Here's how the part is built. I have some questions about the finished solid (model axes, mm). A direction names the side the tool comes from. Round coordinates to 2 decimals unless told otherwise and drop trailing zeros. Order: outer loops, then holes, each group sorted by start corner. A loop starts at its lowest first (then second) coordinate and runs counter-clockwise, first axis right, second up. Notation, with made-up numbers: (87.5, 73) -> (145.5, 73) arc R25 ccw to (145.5, 99) -> close; hole circle Ø1 at (43, 15). An arc over 180 degrees is marked (long way). Use a Markdown table: item, result. Add a question column.
(1) Thinking about a two-plate mould opening in X: for faces 6 (the face through (10, 19, 0)), 7 (the face through (0, 34, 20.25)), 8 (the face through (-0.6, 31, -23)), 9 (the face through (-5, 29, -22)), which applies, pulls with the +X half, pulls with the -X half, needs draft (parallel to the pull), parting line crosses it, or undercut?
(2) I want a section at A-A, the plane z = -24.25. Please give me the cut outline in (x, y), then the cut area to 3 significant figures.
(3) I'm going to push flat-ended pins straight in: P1, Ø0.6, axis at y = 30.5, z = -24.5, coming from the +X side; P2, Ø4, axis at y = 6, z = 23.5, coming from the +X side; P3, Ø4, axis at x = 0, z = 10.25, coming from the +Y side; P4, Ø5, axis at x = 4, z = -22, coming from the -Y side. Where does each tip first touch, or does it pass through?
(4) I want a section at C-C, the plane x = 0. Please give me the cut outline in (y, z), then the cut area to 3 significant figures.
(5) If I drill on probe 1 along X at (y, z) = (29, -24); probe 2 along Z at (x, y) = (5, 28.6); probe 3 along Y at (x, z) = (8.25, -20.5), over which ranges is the centre line in solid material (lowest first)?
(6) I want a section at B-B, the plane z = 10.25. Please give me the cut outline in (x, y).
(7) On a 3-axis mill with a long thin cutter (end or side, diameter ignored), from which of +Z, -Z, +X, -X, +Y, -Y can I reach the whole of each face in a straight line? I mean faces 1 (the face through (0, 8, 23)), 2 (the face through (0, 27.5, -24)), 3 (the face through (6, 30, 22)), 4 (the face through (-6, 30, -22)), 5 (the face through (-3.75, 6, 23)). Say none if no direction works.
(8) I want a section at D-D, the plane y = 31. Please give me the cut outline in (x, z), then the cut area to 3 significant figures.
Autodesk Inventor part; units mm, degrees
ref_plane "YZ Plane" through (0, 0, 0) normal (1, 0, 0) x (0, 1, 0)
ref_plane "XZ Plane" through (0, 0, 0) normal (0, 1, 0) x (-1, 0, 0)
ref_plane "XY Plane" through (0, 0, 0) normal (0, 0, 1) x (1, 0, 0)
sketch "Sketch1" plane through (0, 0, 0) normal (0, 1, 0) x (-1, 0, 0)
  line L0 (-10, 20.25) -> (10, 20.25)
  line L1 (10, 20.25) -> (10, -20.25)
  line L2 (10, -20.25) -> (-10, -20.25)
  line L3 (-10, -20.25) -> (-10, 20.25)
  point P0 (0, 0)
  point P1 (0, 20.25)
  point P2 (10, 0)
  dimension "s_width" = 40.5
  dimension "s_depth" = 20
extrude "Extrusion1" add sketch "Sketch1" along normal blind 38
sketch "Sketch2" plane through (-10, 0, 20.25) normal (0, 0, 1) x (1, 0, 0)
  line L0 (0, 38) -> (20, 38) construction
  line L1 (10, 38) -> (10, 0) construction
  line L2 (0, 27.5) -> (20, 27.5)
  line L3 (20, 27.5) -> (20, 30)
  line L4 (20, 30) -> (0, 30)
  line L5 (0, 30) -> (0, 27.5)
  dimension "s_land_thickness" = 2.5
  dimension "s_land_dist_top" = 8
extrude "Extrusion2" add sketch "Sketch2" along normal blind 6.5 and the other way blind 47
sketch "Sketch3" plane through (-10, 30, 20.25) normal (0, 1, 0) x (1, 0, 0)
  line L0 (0, -6.5) -> (0, 0) construction
  line L1 (20, 0) -> (20, -6.5) construction
  circle A0 centre (5, -4) radius 2.25
  line L2 (0, -4) -> (20, -4) construction
  line L3 (20, -6.5) -> (0, -6.5)
  line L4 (0, 47) -> (0, 40.5) construction
  line L5 (0, 44.5) -> (20, 44.5) construction
  line L6 (20, 47) -> (20, 40.5) construction
  line L7 (0, 47) -> (20, 47)
  circle A1 centre (15, 44.5) radius 2.25
  circle A2 centre (15, -4) radius 2.25
  circle A3 centre (5, 44.5) radius 2.25
  point P0 (10, 20.25)
  dimension "s_hole_dia" = 4.5
  dimension "s_hole_front_dist" = 2.5
  dimension "d13" = 2.5
  dimension "s_hole_side_dist" = 2.75
  dimension "d42" = 2.75
extrude "Extrusion3" cut sketch "Sketch3" against normal up to next
sketch "Sketch4" plane through (-10, 0, 20.25) normal (0, 0, 1) x (1, 0, 0)
  line L0 (6.25, 3) -> (13.75, 3)
  line L1 (13.75, 3) -> (13.75, 8)
  line L2 (13.75, 8) -> (6.25, 8)
  line L3 (6.25, 8) -> (6.25, 3)
  line L4 (10, 0) -> (10, 27.5) construction
  line L5 (20, 27.5) -> (0, 27.5) construction
  line L6 (20, 0) -> (0, 0) construction
  point P0 (10, 8)
  dimension "s_cable_height" = 5
  dimension "s_cable_width" = 7.5
  dimension "s_cable_dist_bottom" = 3
extrude "Extrusion4" add sketch "Sketch4" along normal blind 6.5
sketch "Sketch5" plane through (-10, 38, 20.25) normal (0, 0, 1) x (1, 0, 0)
  line L0 (0, 0) -> (20, 0) construction
  line L1 (10, 0) -> (10, -8) construction
  line L2 (0, -8) -> (20, -8) construction
  line L3 (0, -8) -> (0, 0) construction
  line L4 (0, -4) -> (20, -4) construction
  line L5 (20, -8) -> (20, 0) construction
  line L6 (9.4, -8) -> (10.6, -8)
  line L7 (10.6, -8) -> (10.6, -6)
  line L8 (10.6, -6) -> (9.4, -6)
  line L9 (9.4, -6) -> (9.4, -8)
  line L10 (20, -8) -> (0, -8)
  point P0 (10, -38)
  point P1 (10, -8)
  dimension "s_land_pin_thickness" = 2
  dimension "d27" = 1.2
extrude "Extrusion5" add sketch "Sketch5" against normal up to surface (53.5 mm away) from surface at 6.5
sketch "Sketch6" plane through (0, 38, 0) normal (0, 1, 0) x (1, 0, 0)
  circle A0 centre (0, -10.25) radius 4.5
  line L0 (0, 0) -> (0, -26.75) construction
  line L1 (-10, -26.75) -> (10, -26.75) construction
  line L2 (10, 20.25) -> (-10, 20.25)
  line L3 (-10, -20.25) -> (10, -20.25)
  dimension "s_shaft_dia" = 9
  dimension "s_shaft_front_dist" = 10
extrude "Extrusion6" add sketch "Sketch6" along normal blind 6
sketch "Sketch8" plane through (0, 44, 10.25) normal (0, 1, 0) x (1, 0, 0)
  circle A0 centre (0, 0) radius 2.5
  circle A1 centre (0, 0) radius 4.5 construction
  point P0 (0, 10.25)
  dimension "d39" = 5
extrude "Extrusion8" cut sketch "Sketch8" against normal blind 12
equation "\"d7\" = s_land + s_width"
equation "\"d13\" = s_hole_front_dist"
equation "\"d42\" = s_hole_side_dist"
properties part number "Servo"
Taken from the geometry:
| question | item | result |
|---|---|---|
| 1 | face 6 | pulls with the +X half |
| 1 | face 7 | needs draft |
| 1 | face 8 | pulls with the -X half |
| 1 | face 9 | undercut |
| 2 | outline | (-10, 27.5) -> (-7.25, 27.5) -> (-7.25, 30) -> (-10, 30) -> close; (-2.75, 27.5) -> (2.75, 27.5) -> (2.75, 30) -> (0.6, 30) -> (0.6, 32) -> (-0.6, 32) -> (-0.6, 30) -> (-2.75, 30) -> close; (7.25, 27.5) -> (10, 27.5) -> (10, 30) -> (7.25, 30) -> close |
| 2 | area | 29.9 mm2 |
| 3 | P1 | stops at x = 0.6 |
| 3 | P2 | stops at x = 3.75 |
| 3 | P3 | stops at y = 32 |
| 3 | P4 | stops at y = 0 |
| 4 | outline | (0, -20.25) -> (27.5, -20.25) -> (27.5, -26.75) -> (32, -26.75) -> (32, -20.25) -> (38, -20.25) -> (38, 5.75) -> (44, 5.75) -> (44, 7.75) -> (32, 7.75) -> (32, 12.75) -> (44, 12.75) -> (44, 14.75) -> (38, 14.75) -> (38, 20.25) -> (32, 20.25) -> (32, 26.75) -> (27.5, 26.75) -> (27.5, 20.25) -> (8, 20.25) -> (8, 26.75) -> (3, 26.75) -> (3, 20.25) -> (0, 20.25) -> close |
| 4 | area | 1,620 mm2 |
| 5 | probe 1 | x = -10 to -7.24, -2.76 to 2.76, 7.24 to 10 |
| 5 | probe 2 | z = -26.75 to -26.5, -22 to 22, 26.5 to 26.75 |
| 5 | probe 3 | y = 27.5 to 30 |
| 6 | outline | (-10, 0) -> (10, 0) -> (10, 38) -> (4.5, 38) -> (4.5, 44) -> (2.5, 44) -> (2.5, 32) -> (-2.5, 32) -> (-2.5, 44) -> (-4.5, 44) -> (-4.5, 38) -> (-10, 38) -> close |
| 7 | face 1 | +Z, +X, -X |
| 7 | face 2 | -Z, +X, -X, -Y |
| 7 | face 3 | +Z, +X, +Y |
| 7 | face 4 | -Z, -X, +Y |
| 7 | face 5 | +Z, -X, -Y |
| 8 | outline | (-10, -20.25) -> (-0.6, -20.25) -> (-0.6, -26.75) -> (0.6, -26.75) -> (0.6, -20.25) -> (10, -20.25) -> (10, 20.25) -> (0.6, 20.25) -> (0.6, 26.75) -> (-0.6, 26.75) -> (-0.6, 20.25) -> (-10, 20.25) -> close |
| 8 | area | 826 mm2 |
